Can you work these out from the model? Positions are in its coordinate system, mm. A direction names the side the tool comes from. Give positions to 0.01 mm unless a question says otherwise; leave off trailing zeros.
1. I'm going to push flat-ended pins straight in: pin 1 (1.8 mm diameter, centred on x = -18, z = 27, fed in from +Y); pin 2 (3 mm diameter, centred on x = -5.5, y = 1.5, fed in from +Z); pin 3 (1.5 mm diameter, centred on y = 2, z = -2, fed in from +X). Where does each tip first touch, or does it pass through?
2. If I drill on probe 1 along Z at (x, y) = (-10.5, 0.4); probe 2 along Z at (x, y) = (-12.5, 0.4) (3 decimals); probe 3 along X at (y, z) = (3.3, 22), over which ranges is the centre line in solid material (lowest first)?
3. Suppose I cut it at A-A (y = 1.6). Give the number of separate pieces and of enclosed holes in the cut face, and give its area (3 significant figures).
4. On a 3-axis mill with a long thin cutter (end or side, diameter ignored), from which of +Z, -Z, +X, -X, +Y, -Y can I reach the whole of each face in a straight line? I mean faces 4 (the cylindrical face through (-14.854, 1.516, 26.825)), 5 (the cylindrical face through (-14.994, 0.419, 27.454)). Say none if no direction works.
5. Thinking about a two-plate mould opening in Z: for faces 1 (the flat face through (-15.587, 1.066, 28.167)), 2 (the flat face through (-7, 0, 13)), 3 (the flat face through (-20.6, 0.85, 26.2)), which applies, pulls with the +Z half, pulls with the -Z half, needs draft (parallel to the pull), parting line crosses it, or undercut?
```python
from build123d import *

# Parameters (mm, degrees)
EXTRUDE_1_DEPTH     = 5
CUT_EXTRUDE_3_DEPTH = 36.932997264
SKETCH_6_R          = 0.65
CUT_EXTRUDE_4_DEPTH = 37.508731303
SKETCH_7_R          = 1.25
CUT_EXTRUDE_5_DEPTH = 0.85
EXTRUDE_2_DEPTH     = 2.837273549
EXTRUDE_3_DEPTH     = 2.162726451
EXTRUDE_4_DEPTH     = 2.837273549


with BuildPart() as part:
    # 草图1 → 凸台-拉伸1 (new body)
    with BuildSketch(Plane(origin=(0, 0, 0), x_dir=(1, 0, 0), z_dir=(0, 1, 0))):
        with BuildLine():
            Line((-11.532787565, -27.66331715), (-19.756338957, -28.685777545))
            ThreePointArc((-19.756338957, -28.685777545), (-21.987823516, -26.947825687), (-20.249871658, -24.716341127))
            Line((-20.249871658, -24.716341127), (-12.48156417, -23.75048266))
            add(Edge.make_bspline(
                [(-12.48156417, -23.75048266), (-12.295612378, -23.67796581), (-11.920949946, -23.514760542), (-11.264517505, -23.162027697), (-10.551390656, -22.655406839), (-9.837584569, -21.94614323), (-9.026907466, -20.848225864), (-8.238987931, -19.16416179), (-7.602196611, -16.706089731), (-7.189047715, -13.934273469), (-6.893621745, -11.087804415), (-6.772952472, -8.470611277), (-6.854171877, -5.379387305), (-7.367845034, -2.192874406), (-8.514649439, 0.65647794), (-9.829040758, 2.401950035), (-11.094940182, 3.531874214), (-11.819819389, 4.028598999), (-12.191592735, 4.253212063)],
                knots=[0.005238239, 0.005238239, 0.005238239, 0.005238239, 0.020781392, 0.036324544, 0.067410849, 0.098497154, 0.129583459, 0.191756069, 0.253928679, 0.316101289, 0.3782739, 0.44044651, 0.50261912, 0.62696434, 0.75130956, 0.87565478, 0.93782739, 1, 1, 1, 1], degree=3))
            ThreePointArc((-12.191592735, 4.253212063), (-12.869192539, 6.999274426), (-10.123130176, 7.67687423))
            add(Edge.make_bspline(
                [(-11.532787565, -27.66331715), (-11.470532884, -27.640873613), (-11.355102626, -27.59953383), (-11.051609278, -27.488475951), (-10.551343717, -27.286553928), (-9.584901148, -26.829408766), (-7.854575968, -25.725812711), (-5.96542891, -23.675110376), (-4.556446234, -20.819990637), (-3.731942919, -17.796654668), (-3.257587757, -14.742999785), (-2.927918963, -11.698935156), (-2.772480823, -8.76409887), (-2.841981487, -5.204938932), (-3.425083428, -1.318171114), (-4.918570201, 2.52848265), (-7.182233346, 5.575301279), (-9.090959394, 7.05327105), (-10.123130176, 7.67687423)],
                knots=[-0.004411621, -0.004411621, -0.004411621, -0.004411621, -0.000488138, 0.003435345, 0.011282311, 0.026976242, 0.058364105, 0.121139832, 0.183915558, 0.246691284, 0.309467011, 0.372242737, 0.435018463, 0.49779419, 0.623345642, 0.748897095, 0.874448547, 1, 1, 1, 1], degree=3))
        make_face()
    extrude(amount=EXTRUDE_1_DEPTH)

    # 草图5 → 切除-拉伸3 (cut, through all)
    with BuildSketch(Plane.XY.offset(20)):
        Polygon((-22.003105308, 4.162726451), (-22.003105308, 5), (-10.276836703, 5), (-10.276836703, 4.162726451), (-10.276836703, 2.162726451), (-22.003105308, 2.162726451), align=None)
    extrude(amount=CUT_EXTRUDE_3_DEPTH, mode=Mode.SUBTRACT)

    # 草图6 → 切除-拉伸4 (cut, through all)
    with BuildSketch(Plane(origin=(0, 5, 0), x_dir=(1, 0, 0), z_dir=(0, 1, 0))):
        with Locations(Location((-20.021110813, -26.759262863, 0), (0, 0, 270))):
            Circle(SKETCH_6_R)
        with Locations(Location((-15.048958849, -26.204756434, 0), (0, 0, 270))):
            Circle(SKETCH_6_R)
    extrude(amount=-CUT_EXTRUDE_4_DEPTH, mode=Mode.SUBTRACT)

    # 草图7 → 切除-拉伸5 (cut)
    with BuildSketch(Plane.XZ):
        with Locations(Location((-20.021110813, 26.759262863, 0), (0, 0, 270))):
            Circle(SKETCH_7_R)
        with Locations(Location((-15.048958849, 26.204756434, 0), (0, 0, 270))):
            Circle(SKETCH_7_R)
    extrude(amount=-CUT_EXTRUDE_5_DEPTH, mode=Mode.SUBTRACT)

    # 草图8 → 凸台-拉伸2 (add)
    with BuildSketch(Plane(origin=(0, 2.162726451, 0), x_dir=(1, 0, 0), z_dir=(0, 1, 0))):
        with BuildLine():
            Line((-12.48156417, -23.75048266), (-12.580826815, -23.920103142))
            ThreePointArc((-12.580826815, -23.920103142), (-10.558019351, -25.323434722), (-11.429255903, -27.626049851))
            add(Edge.make_bspline(
                [(-11.429255903, -27.626049851), (-11.402483913, -27.616408571), (-11.312274879, -27.583861794), (-11.051609278, -27.488475951), (-10.694139024, -27.344190351), (-10.414634593, -27.218588376), (-10.276836703, -27.153356774)],
                knots=[-0.002196957, -0.002196957, -0.002196957, -0.002196957, -0.000488138, 0.003435345, 0.011282311, 0.019136837, 0.019136837, 0.019136837, 0.019136837], degree=3))
            Line((-10.276836703, -27.153356774), (-10.276836703, -22.371362309))
            add(Edge.make_bspline(
                [(-10.276836703, -22.371362309), (-10.372821557, -22.463117226), (-10.724386033, -22.778306526), (-11.264517505, -23.162027697), (-11.920949946, -23.514760542), (-12.295612378, -23.67796581), (-12.48156417, -23.75048266)],
                knots=[0.925593927, 0.925593927, 0.925593927, 0.925593927, 0.93782739, 0.968913695, 0.984456847, 1, 1, 1, 1], degree=3))
        make_face()
    extrude(amount=EXTRUDE_2_DEPTH)

    # 草图9 → 凸台-拉伸3 (add)
    with BuildSketch(Plane.XZ):
        with BuildLine():
            Line((-20.489918003, 24.746186856), (-12.48156417, 23.75048266))
            add(Edge.make_bspline(
                [(-12.48156417, 23.75048266), (-12.295612378, 23.67796581), (-11.920949946, 23.514760542), (-11.264517505, 23.162027697), (-10.551390656, 22.655406839), (-9.837584569, 21.94614323), (-9.026907466, 20.848225864), (-8.238987931, 19.16416179), (-7.602196611, 16.706089731), (-7.189047715, 13.934273469), (-6.987988897, 11.997044646), (-6.917012362, 11.050106293), (-6.91422073, 11.012251503)],
                knots=[0.005238239, 0.005238239, 0.005238239, 0.005238239, 0.020781392, 0.036324544, 0.067410849, 0.098497154, 0.129583459, 0.191756069, 0.253928679, 0.316101289, 0.3782739, 0.380867603, 0.380867603, 0.380867603, 0.380867603], degree=3))
            add(Edge.make_bspline(
                [(-20.489918003, 24.746186856), (-9.085568026, 22.00342521), (-6.91422073, 11.012251503)],
                knots=[0, 0, 0, 1, 1, 1], degree=2))
        make_face()
    extrude(amount=-EXTRUDE_3_DEPTH)

    # 草图10 → 凸台-拉伸4 (add)
    with BuildSketch(Plane(origin=(0, 2.162726451, 0), x_dir=(1, 0, 0), z_dir=(0, 1, 0))):
        with BuildLine():
            Line((-12.48156417, -23.75048266), (-12.573747328, -23.90800568))
            add(Edge.make_bspline(
                [(-12.573747328, -23.90800568), (-13.049488997, -23.93391524), (-14.700965999, -23.963867562), (-16.426938548, -23.94912182), (-15.35263855, -22.852847317)],
                knots=[0, 0, 0, 0, 0.570111163, 1, 1, 1, 1], degree=3))
            add(Edge.make_bspline(
                [(-15.35263855, -22.852847317), (-8.541278489, -19.248278275), (-6.91422073, -11.012251503)],
                knots=[0, 0, 0, 1, 1, 1], degree=2))
            add(Edge.make_bspline(
                [(-6.91422073, -11.012251503), (-6.917012362, -11.050106293), (-6.987988897, -11.997044646), (-7.189047715, -13.934273469), (-7.602196611, -16.706089731), (-8.238987931, -19.16416179), (-9.026907466, -20.848225864), (-9.837584569, -21.94614323), (-10.551390656, -22.655406839), (-11.264517505, -23.162027697), (-11.920949946, -23.514760542), (-12.295612378, -23.67796581), (-12.48156417, -23.75048266)],
                knots=[0.624370637, 0.624370637, 0.624370637, 0.624370637, 0.62696434, 0.68913695, 0.75130956, 0.81348217, 0.87565478, 0.906741085, 0.93782739, 0.968913695, 0.984456847, 1, 1, 1, 1], degree=3))
        make_face()
    extrude(amount=EXTRUDE_4_DEPTH)


solid = part.part
```
Checks:
1. pin 1: stops at y = 2.16
1. pin 2: stops at z = 24.73
1. pin 3: stops at x = -4.48
2. probe 1: z = -7.85 to -2.99, 18.95 to 27.26
2. probe 2: z = -7.447 to -4.483, 20.955 to 27.784
2. probe 3: x = -13.91 to -5.17
3. separate pieces: 1
3. enclosed holes: 2
3. area: 215 mm2
4. face 4: +Y, -Y
4. face 5: -Y
5. face 1: pulls with the +Z half
5. face 2: needs draft
5. face 3: undercut
